```python
from build123d import *

# Parameters (mm, degrees)
F0_R          = 25.91
F1_DEPTH      = 7
F1_DEPTH_BACK = 7
F2_R          = 17
F3_DEPTH      = 7
F3_DEPTH_BACK = 7
F6_START      = -6
F5_W          = 8
F5_H          = 14
F6_DEPTH      = 14
F7_R          = 2.15
F8_DEPTH      = 30
F8_DEPTH_BACK = 30
F9_W          = 10
F9_H          = 14
F10_DEPTH     = 10
F14_W         = 122.705668211
F14_H         = 84.9680826068
F15_DEPTH     = 18


with BuildPart() as f1:
    # F0 (on Front) → F1 (new body, two sides)
    with BuildSketch(Plane.XZ) as f1_sk:
        Circle(F0_R)
    extrude(amount=F1_DEPTH)
    extrude(f1_sk.sketch, amount=-F1_DEPTH_BACK)

    # F2 (on Front) → F3 (cut, two sides)
    with BuildSketch(Plane.XZ) as f3_sk:
        Circle(F2_R)
    extrude(amount=-F3_DEPTH, mode=Mode.SUBTRACT)
    extrude(f3_sk.sketch, amount=F3_DEPTH_BACK, mode=Mode.SUBTRACT)

    # F5 (on face) → F6 (join)
    with BuildSketch(Plane.XY.offset(F6_START)):
        with Locations((-19.91, 0)):
            Rectangle(F5_W, F5_H)
        with Locations((19.91, 0)):
            Rectangle(F5_W, F5_H)
    extrude(amount=-F6_DEPTH)

    # F7 (on face) → F8 (cut, two sides)
    with BuildSketch(Plane.XY) as f8_sk:
        with Locations((-19.1982129737, 0)):
            Circle(F7_R)
        with Locations((19.0490627756, 0)):
            Circle(F7_R)
    extrude(amount=F8_DEPTH, mode=Mode.SUBTRACT)
    extrude(f8_sk.sketch, amount=-F8_DEPTH_BACK, mode=Mode.SUBTRACT)

    # F9 (on face) → F10 (cut)
    with BuildSketch(Plane(origin=(0, 0, -20), x_dir=(1, 0, 0), z_dir=(0, 0, -1))):
        with Locations((-18.91, 0)):
            Rectangle(F9_W, F9_H)
        with Locations((18.91, 0)):
            Rectangle(F9_W, F9_H)
    extrude(amount=F10_DEPTH, mode=Mode.SUBTRACT)

    # F14 (on 3pt) → F15 (cut)
    with BuildSketch(Plane(origin=(0, 0, 11.36), x_dir=(1, 0, 0), z_dir=(0, 0, -1))):
        with Locations((8.9623853564, -3.6773085594)):
            Rectangle(F14_W, F14_H)
    extrude(amount=-F15_DEPTH, mode=Mode.SUBTRACT)


solid = f1.part
```
Design review of the part built by this model. Coordinates are the model's own, in mm. A direction names the side the tool comes from. Give positions to 0.01 mm unless a question says otherwise; leave off trailing zeros. Loops run counter-clockwise (first coordinate to the right, second up) from the corner with the lowest first, then second, coordinate; pieces in that order, holes last. Notation, with made-up numbers: M -12,72.25 L 29,72.25 A12 ccw 29,85.25 Z; hole C -17,-31 d7. An arc over 180 degrees is marked long. Return JSON: item names as keys, results as strings. Group by question number.
Item 1: Tool access review of faces 5 (the flat face through (-23.91, 0, -15)), 6 (the cylindrical face through (25.903, -0.098, 0.602)), 7 (the flat face through (23.91, 0, -15)): name each direction out of +Z, -Z, +X, -X, +Y, -Y from which nothing blocks a thin tool from reaching the whole face with its end or side.
Item 2: Insertion check: pin 1 Ø0.6 at (y, z) = (-1, -21.5) entering from -X; pin 2 Ø5 at (x, y) = (21.5, -2) entering from -Z; pin 3 Ø2 at (x, y) = (10.5, -0.5) entering from +Z; pin 4 Ø5.5 at (x, y) = (-19.2, 0) entering from +Z. Each pin has a flat end and moves straight along its axis. Give the tip position at first contact, or say it passes through.
Item 3: We need section C-C (z = 0). Give the boundary of the cut face in (x, y), and give its area (3 significant figures).
Item 4: For probe 1 along X at (y, z) = (-1, 4.5); probe 2 along Z at (x, y) = (-20, 6); probe 3 along X at (y, z) = (4, -1.5), list the stretches that pass through material, from the lowest coordinate up.
Item 5: We need section D-D (y = 4.25). Give the boundary of the cut face in (x, z), and give its area (3 significant figures).
Item 6: Mouldability with a two-part tool opening along X and no side actions: class faces 1 (the cylindrical face through (-25.894, -0.098, 0.91)), 2 (the cylindrical face through (21.1, 0.65, -4.1)), 3 (the flat face through (0, 7, -19)), 4 (the cylindrical face through (-21.346, 0.095, -4.1)) as released by +X, released by -X, zero draft, split by the parting line, or undercut.
Item 7: We need section B-B (y = -1). Give the boundary of the cut face in (x, z), and give its area (3 significant figures).
Item 8: We need section A-A (z = -15). Give the boundary of the cut face in (x, y), and give its area (3 significant figures).
Output:
{
 "1": {"face 5": "-Z, -X, +Y, -Y", "face 6": "+X, +Y, -Y", "face 7": "-Z, +X, +Y, -Y"},
 "2": {"pin 1": "stops at x = -13.91", "pin 2": "stops at z = -20", "pin 3": "stops at z = -12.52", "pin 4": "stops at z = 11.36"},
 "3": {"outline": "M -25.91,-7 L -17,-7 L -17,7 L -25.91,7 Z; M 17,-7 L 25.91,-7 L 25.91,7 L 17,7 L 17,0.65 A2.15 cw long 17,-0.65 Z; hole C -19.2,0 d4.3", "area": "221 mm^2"},
 "4": {"probe 1": "x = -25.52 to -21.1, -17.29 to -16.39, 16.39 to 17.15, 20.95 to 25.52", "probe 2": "z = -20 to 11.36", "probe 3": "x = -25.87 to -16.93, 16.93 to 25.87"},
 "5": {"outline": "M -23.91,-20 L -13.91,-20 L -13.91,-21.86 A25.91 ccw 13.91,-21.86 L 13.91,-20 L 23.91,-20 L 23.91,-9.98 A25.91 ccw 23.29,11.36 L 12.65,11.36 A17 cw long -12.65,11.36 L -23.29,11.36 A25.91 ccw -23.91,-9.98 Z", "area": "871 mm^2"},
 "6": {"face 1": "released by -X", "face 2": "undercut", "face 3": "zero draft", "face 4": "undercut"},
 "7": {"outline": "M -23.91,-20 L -21.1,-20 L -21.1,11.36 L -23.29,11.36 A25.91 ccw -23.91,-9.98 Z; M -17.29,-20 L -13.91,-20 L -13.91,-21.86 A25.91 ccw 13.91,-21.86 L 13.91,-20 L 17.15,-20 L 17.15,11.36 L 12.65,11.36 A17 cw long -12.65,11.36 L -17.29,11.36 Z; M 20.95,-20 L 23.91,-20 L 23.91,-9.98 A25.91 ccw 23.29,11.36 L 20.95,11.36 Z", "area": "633 mm^2"},
 "8": {"outline": "M -23.91,-7 L -8,-7 L -8,7 L -23.91,7 Z; M 8,-7 L 23.91,-7 L 23.91,7 L 8,7 Z; hole C -19.2,0 d4.3; hole C 19.05,0 d4.3", "area": "416 mm^2"}
}
